The model under review builds one solid part; all positions refer to its coordinate system, in mm. Face numbers are marked on the shaded views. A direction names the side the tool comes from. Coordinates: 2 decimals unless noted, no trailing zeros. Loops run counter-clockwise (first coordinate to the right, second up) from the corner with the lowest first, then second, coordinate; pieces in that order, holes last. Notation, with made-up numbers: (6.5, 11) - (32.5, 11) arc R27 cw to (32.5, 47) - close; hole circle Ø4 at (62.25, 33.25). An arc over 180 degrees is marked (long way). One line per item, written item: value. Start each with the question number.
1. We need section D-D, the plane z = -1. Give the boundary of the cut face in (x, y) (3 decimals).
2. Insertion check: P1, Ø1.1, axis at y = 1, z = 4, coming from the -X side; P2, Ø0.8, axis at y = 1, z = -2, coming from the -X side. Each pin has a flat end and moves straight along its axis. Give the tip position at first contact, or say it passes through.
3. To check wall thickness, follow line 1 (Z direction, x = 10.75, y = 1.25); line 2 (Z direction, x = 15.24, y = 0.8); line 3 (Z direction, x = 10, y = 1.1). State the ranges of each line that lie inside material, in increasing order.
4. For the marked faces 1, 2 and 3, list the 3-axis set-ups (+Z, -Z, +X, -X, +Y, -Y) from which the entire face can be reached by the end or side of a thin tool; tool diameter is ignored.
5. We need section B-B, the plane y = 2.5. Give the boundary of the cut face in (x, z) (3 decimals).
6. We need section A-A, the plane z = 7.75. Give the boundary of the cut face in (x, y) (3 decimals), then the cut area to 3 significant figures.
7. We need section C-C, the plane x = 21.25. Give the boundary of the cut face in (y, z) (3 decimals), then the cut area to 3 significant figures.
8. Mouldability with a two-part tool opening along X and no side actions: class the marked faces 4, 5, 6 and 7 as +X half, -X half, draft (parallel to the pull), parting line (faces both ways), or undercut.
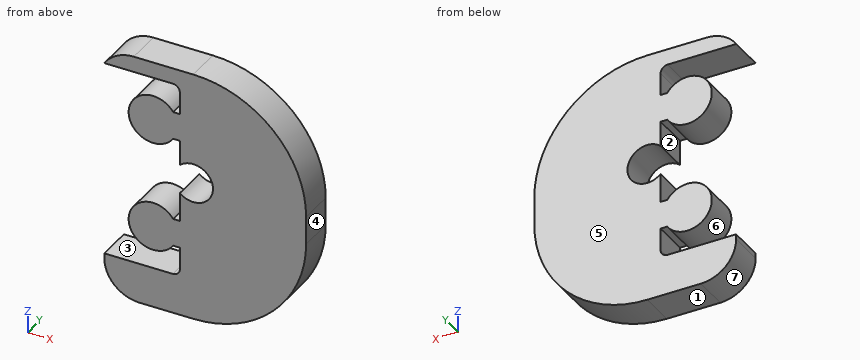
from build123d import *

# Parameters (mm, degrees)
SKETCH1_W           = 50.8
SKETCH1_H           = 22.86
BOSS_EXTRUDE1_DEPTH = 3.175
FILLET1_R           = 10.16
SKETCH3_R           = 1.778
CUT_EXTRUDE1_DEPTH  = 29.033649869
FILLET3_R           = 10.16
CUT_EXTRUDE3_DEPTH  = 29.033649869
FILLET4_R           = 0.635
FILLET5_R           = 3.175


with BuildPart() as part:
    # Sketch1 → Boss-Extrude1 (new body)
    with BuildSketch(Plane(origin=(0, 0, 0), x_dir=(1, 0, 0), z_dir=(0, 1, 0))):
        Rectangle(SKETCH1_W, SKETCH1_H)
    extrude(amount=BOSS_EXTRUDE1_DEPTH)

    # Fillet1
    fillet1_edges = [part.edges().sort_by_distance(p)[0] for p in [
        (25.4, 1.5875, 11.43),
        (-25.4, 1.5875, 11.43),
    ]]
    fillet(fillet1_edges, radius=FILLET1_R)

    # Sketch3 → Cut-Extrude1 (cut, through all)
    with BuildSketch(Plane(origin=(0, 3.175, 0), x_dir=(1, 0, 0), z_dir=(0, 1, 0))):
        with Locations(Location((15.24, -1.27, 0), (0, 0, 270))):
            Circle(SKETCH3_R)
        with Locations(Location((-3.81, -1.27, 0), (0, 0, 270))):
            Circle(SKETCH3_R)
    extrude(amount=-CUT_EXTRUDE1_DEPTH, mode=Mode.SUBTRACT)

    # Fillet3
    fillet3_edges = [part.edges().sort_by_distance(p)[0] for p in [
        (-25.4, 1.5875, -11.43),
        (25.4, 1.5875, -11.43),
    ]]
    fillet(fillet3_edges, radius=FILLET3_R)

    # Sketch5 → Cut-Extrude3 (cut, through all)
    with BuildSketch(Plane.XZ):
        with BuildLine():
            Line((7.239, -11.43), (7.239, -7.799110591))
            Line((7.239, -7.799110591), (14.039031064, -7.799110591))
            Line((14.039031064, -7.799110591), (14.039031064, -5.149110591))
            Line((14.039031064, -5.149110591), (13.439031064, -5.149110591))
            ThreePointArc((13.439031064, -5.149110591), (9.428644365, -3.899110591), (13.439031064, -2.649110591))
            Line((13.439031064, -2.649110591), (14.039031064, -2.649110591))
            Line((14.039031064, -2.649110591), (14.039031064, 4.850889409))
            Line((14.039031064, 4.850889409), (13.439031064, 4.850889409))
            ThreePointArc((13.439031064, 4.850889409), (9.428644366, 6.100889409), (13.439031064, 7.350889409))
            Line((13.439031064, 7.350889409), (14.039031064, 7.350889409))
            Line((14.039031064, 7.350889409), (14.039031064, 10.000889409))
            Line((14.039031064, 10.000889409), (7.239, 10.000889409))
            Line((7.239, 10.000889409), (7.239, 11.43))
            Line((7.239, 11.43), (-25.4, 11.43))
            Line((-25.4, 11.43), (-25.4, -11.43))
            Line((-25.4, -11.43), (7.239, -11.43))
        make_face()
    extrude(amount=-CUT_EXTRUDE3_DEPTH, mode=Mode.SUBTRACT)

    # Fillet4
    fillet4_edges = [part.edges().sort_by_distance(p)[0] for p in [
        (14.039031064, 1.5875, 10.000889409),
        (14.039031064, 1.5875, -7.799110591),
    ]]
    fillet(fillet4_edges, radius=FILLET4_R)

    # Fillet5
    # the kernel refuses this fillet: 3.175 mm, written as the material it takes off along each edge
    with BuildSketch(Plane(origin=(7.239, -7.9375, -11.43), x_dir=(1, 0, 0), z_dir=(0, 1, 0))) as fillet5_piece_1:
        with BuildLine():
            CenterArc((FILLET5_R, -FILLET5_R), FILLET5_R, 90, 90)
            Line((0, -FILLET5_R), (-FILLET5_R * 0.02, -FILLET5_R))
            Line((-FILLET5_R * 0.02, -FILLET5_R), (-FILLET5_R * 0.02, FILLET5_R * 0.02))
            Line((-FILLET5_R * 0.02, FILLET5_R * 0.02), (FILLET5_R, FILLET5_R * 0.02))
            Line((FILLET5_R, FILLET5_R * 0.02), (FILLET5_R, 0))
        make_face()
    extrude(amount=19.05, mode=Mode.SUBTRACT)
    with BuildSketch(Plane(origin=(7.239, -6.629713028, 11.43), x_dir=(1.52265132002689e-12, 0, -1.0), z_dir=(0, 1, 0))) as fillet5_piece_2:
        with BuildLine():
            CenterArc((3.175, -2.651885211), FILLET5_R, 123.359221801, 56.640778199)
            Line((0, -2.651885211), (-0.0635, -2.651885211))
            Line((-0.0635, -2.651885211), (-0.0635, 0))
            Line((-0.0635, 0), (0, 0.0635))
            ThreePointArc((0, 0.0635), (0.714555296, 0.0635), (1.394192803, 0.053037704))
            Line((1.394192803, 0.053037704), (1.429110591, 0))
        make_face()
    extrude(amount=16.434426055, mode=Mode.SUBTRACT)


solid = part.part
Findings below:
1. outline: (14.039, 0) - (25.4, 0) - (25.4, 3.175) - (14.039, 3.175) - close
2. P1: x = 10.07
2. P2: x = 10.02
3. line 1: -11.43 to -7.8, -5.92 to -1.88, 4.08 to 8.12, 10 to 11.43
3. line 2: -11.43 to -0.51, 3.05 to 11.43
3. line 3: -11.4 to -7.8, -5.38 to -2.42, 4.62 to 7.58, 10 to 11.43
4. face 1: -Z, +X, -X, +Y, -Y
4. face 2: +Y, -Y
4. face 3: -X, +Y, -Y
5. outline: (7.239, -8.255) arc R3.175 ccw to (10.414, -11.43) - (15.24, -11.43) arc R10.16 ccw to (25.4, -1.27) - (25.4, 1.27) arc R10.16 ccw to (15.24, 11.43) - (9.891, 11.43) arc R3.175 ccw to (7.239, 10.001) - (13.404, 10.001) arc R0.635 cw to (14.039, 9.366) - (14.039, 7.351) - (13.439, 7.351) arc R2.2 ccw (long way) to (13.439, 4.851) - (14.039, 4.851) - (14.039, 2.581) arc R1.778 cw (long way) to (14.039, -0.041) - (14.039, -2.649) - (13.439, -2.649) arc R2.2 ccw (long way) to (13.439, -5.149) - (14.039, -5.149) - (14.039, -7.164) arc R0.635 cw to (13.404, -7.799) - (7.239, -7.799) - close
6. outline: (10.172, 0) - (13.085, 0) - (13.085, 3.175) - (10.172, 3.175) - close; (14.039, 0) - (23.065, 0) - (23.065, 3.175) - (14.039, 3.175) - close
6. area: 37.9 mm2
7. outline: (0, -9.462) - (3.175, -9.462) - (3.175, 9.462) - (0, 9.462) - close
7. area: 60.1 mm2
8. face 4: +X half
8. face 5: draft
8. face 6: undercut
8. face 7: -X half
